Part print with two shaded views. Sizes in mm from the minimum x, y, z corner. Give positions to 0.01 mm unless a question says otherwise; leave off trailing zeros. Write each loop counter-clockwise with the first axis right and the second up, starting at its lowest first coordinate (ties: lowest second). Pieces come first, ordered by that corner, then holes. Notation, with made-up numbers: (17.5, 15) -> (75.5, 15) arc R12 ccw to (75.5, 36) -> close; hole circle Ø7 at (2, 86.5). An arc over 180 degrees is marked (long way). Use one line per item in the form item = value. Start each with the question number.
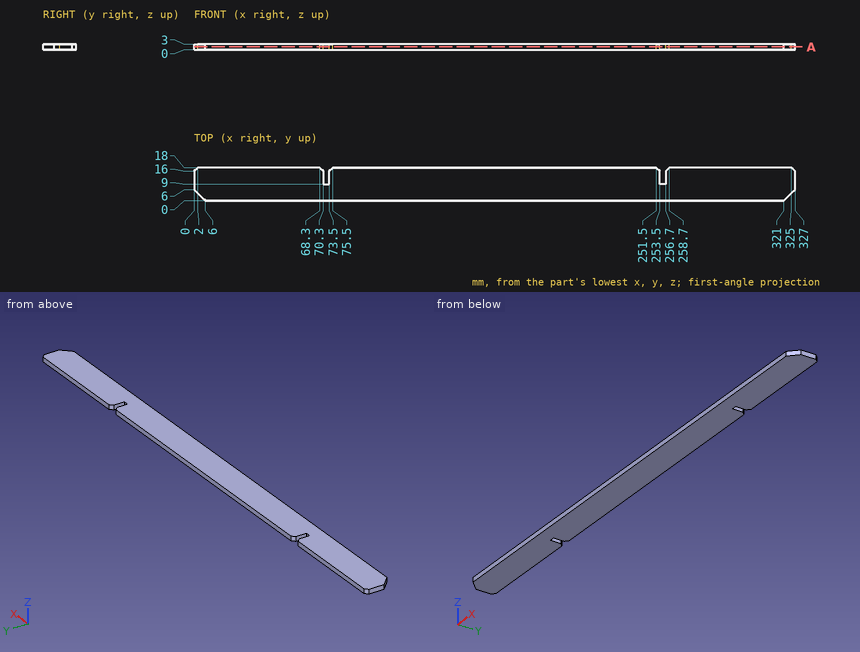
1) Pin check, flat tip, straight feed: pin 1 (1.5 mm diameter, centred on x = 256, z = 1.5, fed in from +Y). Stop position of the tip, or through.
2) Cut at A-A (z = 1.4). Give the cut face in (x, y), and give its area (3 significant figures).
3) Wall check: line 1 along X through (y, z) = (12, 0.9); line 2 along X through (y, z) = (16.25, 2.1); line 3 along X through (y, z) = (5.25, 0.7). Give the ranges that are in metal, low to high. Write a range as from..to.
Final values:
q1.pin_1 = 16.05
q2.outline = (0, 6) -> (6, 0) -> (321, 0) -> (327, 6) -> (327, 16) -> (325, 18) -> (258.7, 18) -> (256.7, 16) -> (256.7, 9) -> (253.5, 9) -> (253.5, 16) -> (251.5, 18) -> (75.5, 18) -> (73.5, 16) -> (73.5, 9) -> (70.3, 9) -> (70.3, 16) -> (68.3, 18) -> (2, 18) -> (0, 16) -> close
q2.area = 5,780 mm^2
q3.line_1 = 0..70.3, 73.5..253.5, 256.7..327
q3.line_2 = 0.25..70.05, 73.75..253.25, 256.95..326.75
q3.line_3 = 0.75..326.25
